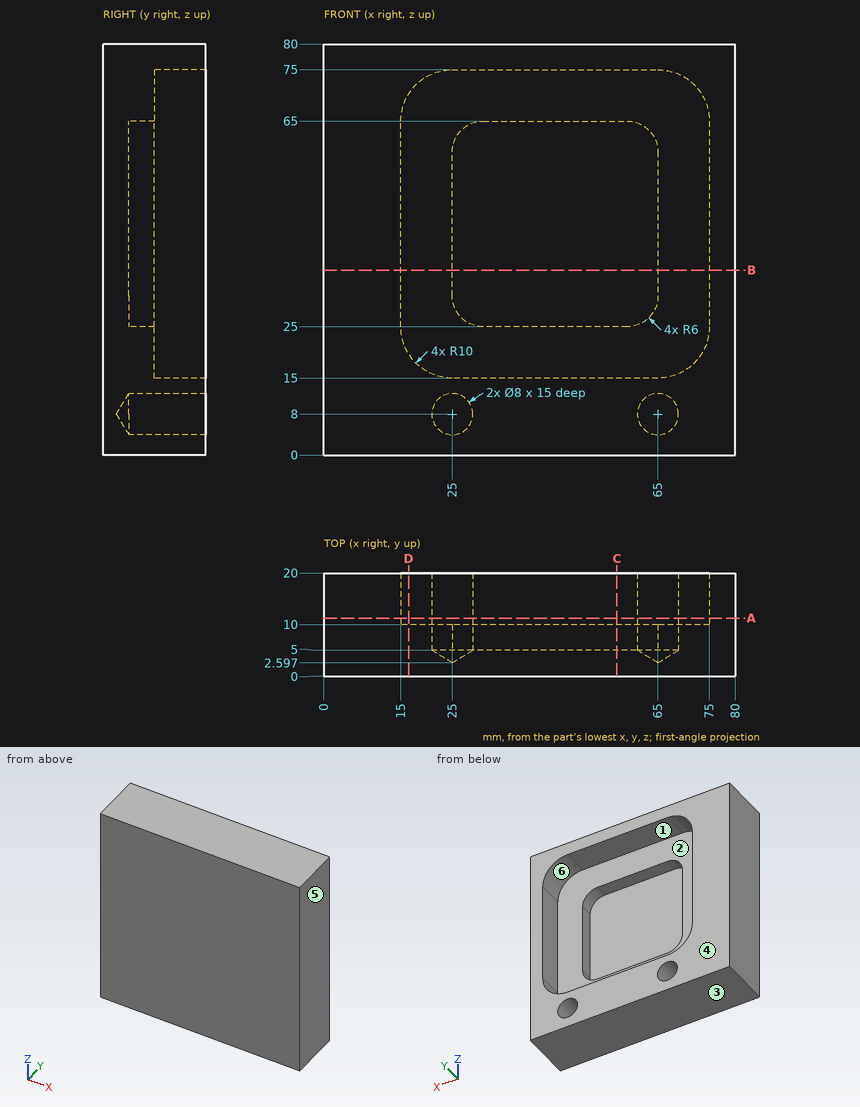
Here's the drawing with two shaded views (mm, measured from the low corner). I have some questions. A direction names the side the tool comes from. Round coordinates to 2 decimals unless told otherwise and drop trailing zeros. Order: outer loops, then holes, each group sorted by start corner. A loop starts at its lowest first (then second) coordinate and runs counter-clockwise, first axis right, second up. Notation, with made-up numbers: M 67.5,56.5 L 97.5,56.5 A18 cw 97.5,81.5 Z; hole C 17.25,52.25 d9. An arc over 180 degrees is marked long. Use CSV: the item, a comma, the result in double quotes.
1) I want a section at B-B (z = 36). List the corners of the cut face in (x, y) for me.
Taken from the geometry:
outline,"M 0,0 L 80,0 L 80,20 L 75,20 L 75,10 L 65,10 L 65,5 L 25,5 L 25,10 L 15,10 L 15,20 L 0,20 Z"
2) I want a section at A-A (y = 11.25). List the corners of the cut face in (x, z) for me.
Taken from the geometry:
outline,"M 0,0 L 80,0 L 80,80 L 0,80 Z; hole M 15,25 A10 ccw 25,15 L 65,15 A10 ccw 75,25 L 75,65 A10 ccw 65,75 L 25,75 A10 ccw 15,65 Z; hole C 25,8 d8; hole C 65,8 d8"
3) I want a section at C-C (x = 57). List the corners of the cut face in (y, z) for me, then the cut area to 3 significant figures.
Taken from the geometry:
outline,"M 0,0 L 20,0 L 20,15 L 10,15 L 10,25 L 5,25 L 5,65 L 10,65 L 10,75 L 20,75 L 20,80 L 0,80 Z"
area,"800 mm^2"
4) I'm going to push flat-ended pins straight in: P1, Ø12, axis at x = 63.5, z = 47.5, coming from the +Y side; P2, Ø1.5, axis at x = 55, z = 59, coming from the +Y side. Where does each tip first touch, or does it pass through?
Taken from the geometry:
P1,"y = 10"
P2,"y = 5"
5) I want a section at D-D (x = 16.5). List the corners of the cut face in (y, z) for me, then the cut area to 3 significant figures.
Taken from the geometry:
outline,"M 0,0 L 20,0 L 20,19.73 L 10,19.73 L 10,70.27 L 20,70.27 L 20,80 L 0,80 Z"
area,"1,090 mm^2"
6) If we mould it in two halves opening along Z, with no side actions, what happens to the marked faces 1, 2, 3 and 4? For each: pulls with the +Z half, pulls with the -Z half, needs draft (parallel to the pull), parting line crosses it, or undercut.
Taken from the geometry:
face 1,"undercut"
face 2,"undercut"
face 3,"pulls with the -Z half"
face 4,"needs draft"
7) On a 3-axis mill with a long thin cutter (end or side, diameter ignored), from which of +Z, -Z, +X, -X, +Y, -Y can I reach the whole of each face in a straight line? I mean the marked faces 5 and 6. Say none if no direction works.
Taken from the geometry:
face 5,"+Z, -Z, +X, +Y, -Y"
face 6,"+Y"
8) I need wall thicknesses on line 1 along X through (y, z) = (8, 8); line 2 along Z through (x, y) = (65, 14.5); line 3 along X through (y, z) = (15, 53). Which ranges of each line are inside material? Lowest first, please. Write a range as [from, to].
Taken from the geometry:
line 1,"[0, 21], [29, 61], [69, 80]"
line 2,"[0, 4], [12, 15], [75, 80]"
line 3,"[0, 15], [75, 80]"
